Could you check a few things on this model? Use its own coordinates, in mm. A direction names the side the tool comes from. Round coordinates to 2 decimals unless told otherwise and drop trailing zeros. Loops run counter-clockwise (first coordinate to the right, second up) from the corner with the lowest first, then second, coordinate; pieces in that order, holes last. Notation, with made-up numbers: (-26, 25) -> (11, 25) arc R16 ccw to (11, 45) -> close; hole circle Ø1 at (69.25, 87). An arc over 180 degrees is marked (long way). Write each question's results on one line, items separated by ' | '.
from build123d import *

# Parameters (mm, degrees)
EXTRUSION1_DEPTH   = 69
ESQUISSE2_R        = 9.25
BOSS_EXTRU_1_DEPTH = 3
BOSS_EXTRU_2_START = 3
ESQUISSE3_R        = 9.25
BOSS_EXTRU_2_DEPTH = 3
CONG_1_R           = 0.2
COQUE2_START       = 1
COQUE2_DEPTH       = 67
COQUE2_START_2     = -2
COQUE2_2_OUTLINE_R = 8.25
COQUE2_2_DEPTH     = 73


# Read off the part's stored shape, not the designer's step: Coque2
with BuildPart() as part:
    # Esquisse1 → Extrusion1 (new body)
    with BuildSketch(Plane.XY):
        with BuildLine():
            ThreePointArc((-8.53680315, -7.705387205), (-7.567547804, -9.297974269), (-7.249086614, -11.134920635))
            ThreePointArc((-7.249086614, -11.134920635), (0, -18.5), (7.249086614, -11.134920635))
            ThreePointArc((7.249086614, -11.134920635), (7.567547804, -9.297974269), (8.53680315, -7.705387205))
            ThreePointArc((8.53680315, -7.705387205), (0, 11.5), (-8.53680315, -7.705387205))
        make_face()
    extrude(amount=EXTRUSION1_DEPTH)

    # Esquisse2 → Boss.-Extru.1 (add)
    with BuildSketch(Plane.XY.offset(69)):
        Circle(ESQUISSE2_R)
    extrude(amount=BOSS_EXTRU_1_DEPTH)

    # Esquisse3 → Boss.-Extru.2 (add)
    with BuildSketch(Plane(origin=(0, 0, 0), x_dir=(-1, 0, 0), z_dir=(0, 0, -1)).offset(BOSS_EXTRU_2_START)):
        with Locations(Location((0, 0, 0), (0, 0, 180))):
            Circle(ESQUISSE3_R)
    extrude(amount=-BOSS_EXTRU_2_DEPTH)

    # Congé1
    cong_1_edges = [part.edges().sort_by_distance(p)[0] for p in [
        (0, -18.5, 69),
        (7.567547804, -9.297974269, 69),
        (-9.25, 0, 72),
        (-9.25, 0, -3),
        (0, 11.5, 69),
        (7.567547804, -9.297974269, 0),
        (0, -18.5, 0),
        (-7.567547804, -9.297974269, 0),
        (0, 11.5, 0),
        (-7.567547804, -9.297974269, 69),
    ]]
    fillet(cong_1_edges, radius=CONG_1_R)

    # Coque2 outline → Coque2 (cut)
    with BuildSketch(Plane.XY.offset(COQUE2_START)):
        with BuildLine():
            ThreePointArc((7.794472441, -7.035353535), (0, 10.5), (-7.794472441, -7.035353535))
            ThreePointArc((-7.794472441, -7.035353535), (-6.631366027, -8.946458012), (-6.249212598, -11.150793651))
            ThreePointArc((-6.249212598, -11.150793651), (0, -17.5), (6.249212598, -11.150793651))
            ThreePointArc((6.249212598, -11.150793651), (6.631366027, -8.946458012), (7.794472441, -7.035353535))
        make_face()
    extrude(amount=COQUE2_DEPTH, mode=Mode.SUBTRACT)

    # Coque2 2 outline → Coque2 2 (cut)
    with BuildSketch(Plane.XY.offset(COQUE2_START_2)):
        Circle(COQUE2_2_OUTLINE_R)
    extrude(amount=COQUE2_2_DEPTH, mode=Mode.SUBTRACT)


solid = part.part
1) If we mould it in two halves opening along Y, with no side actions, what happens to faces 5 (the cylindrical face through (0.339, 10.495, 34.031)), 6 (the flat face through (1, -10, 0)), 7 (the cylindrical face through (0.371, 11.494, 34.02))? For each: released by +Y, released by -Y, zero draft, split by the parting line, or undercut.
Model answer:
face 5: undercut | face 6: zero draft | face 7: split by the parting line
2) I'm going to push flat-ended pins straight in: pin 1 (5 mm diameter, centred on x = 3, z = 8.5, fed in from -Y); pin 2 (3 mm diameter, centred on y = -2.5, z = 24, fed in from -X); pin 3 (10 mm diameter, centred on y = -12.5, z = 23.5, fed in from +X). Where does each tip first touch, or does it pass through?
Model answer:
pin 1: stops at y = -18.48 | pin 2: stops at x = -11.46 | pin 3: stops at x = 8.72
3) For faces 1 (the cylindrical face through (4.268, 8.206, -1.42)), 2 (the flat face through (0, 0, 72)), 3 (the cylindrical face through (7.62, -3.16, 69.48)), 4 (the flat face through (1, -10, 69)), which set-ups out of +Z, -Z, +X, -X, +Y, -Y let a thin tool reach every point of the face, with its end or its side?
Model answer:
face 1: -Z | face 2: +Z, +X, -X, +Y, -Y | face 3: none | face 4: +Z
4) I want a section at B-B, the plane z = 39. Write out the boundary of the cut face in (x, y), plus the area to 3 significant figures.
Model answer:
outline: (-8.54, -7.71) arc R5 cw to (-7.25, -11.13) arc R7.25 ccw (long way) to (7.25, -11.13) arc R5 cw to (8.54, -7.71) arc R11.5 ccw (long way) to start; hole (-7.79, -7.04) arc R6 cw to (-6.25, -11.15) arc R6.25 ccw (long way) to (6.25, -11.15) arc R6 cw to (7.79, -7.04) arc R10.5 ccw (long way) to start | area: 80.4 mm2
5) I need wall thicknesses on line 1 (X direction, y = 0, z = 28); line 2 (Y direction, x = 0, z = 69.5); line 3 (Z direction, x = 0, y = 10). Which ranges of each line are inside material? Lowest first, please.
Model answer:
line 1: x = -11.5 to -10.5, 10.5 to 11.5 | line 2: y = -9.25 to -8.25, 8.25 to 9.25 | line 3: z = 0 to 1, 68 to 69
